Input: part model. Units: mm. Frame: model coordinates. Face numbers are marked on the shaded views. A direction names the side the tool comes from. Coordinates: 2 decimals unless noted, no trailing zeros. Order: outer loops, then holes, each group sorted by start corner. A loop starts at its lowest first (then second) coordinate and runs counter-clockwise, first axis right, second up. Notation, with made-up numbers: (4.25, -30.75) - (25.25, -30.75) arc R23 ccw to (25.25, 6.25) - close; hole circle Ø7 at (-2, -40). An arc over 180 degrees is marked (long way). Answer as CSV lines item,"result". Start each with the question number.
Item 1: Draft query along X for the marked faces 1, 2, 3 and 4. Return one class per face: +X half, -X half, draft (parallel to the pull), parting line (faces both ways), or undercut.
Item 2: Access query for the marked faces 5, 6 and 7. Directions: +Z, -Z, +X, -X, +Y, -Y. A direction counts if a zero-diameter tool reaches every point of the face in a straight line with its end or side. Return the directions, or none.
Item 3: Section B-B (x = -2). Output: boundary loops of the cut face in (y, z), and give its area (3 significant figures).
Item 4: Section A-A (z = -0.05). Output: boundary loops of the cut face in (x, y) (3 decimals), and give its area (3 significant figures).
Item 5: Material intervals for line 1 along X through (y, z) = (0, -0.5) (3 decimals); line 2 along X through (y, z) = (0, -0.05); line 3 along Y through (x, z) = (-0.7, 0.05) (3 decimals), sorted ascending.
Item 6: First-contact query: pin 1 (1 mm diameter, centred on x = 1.5, z = 1, fed in from -Y); pin 2 (2.5 mm diameter, centred on x = 0, y = 0, fed in from +Z) (3 decimals). Flat tips, straight axial feed; report the tip coordinate or a pass-through.
Item 7: Section C-C (z = 0.8). Output: boundary loops of the cut face in (x, y) (3 decimals).
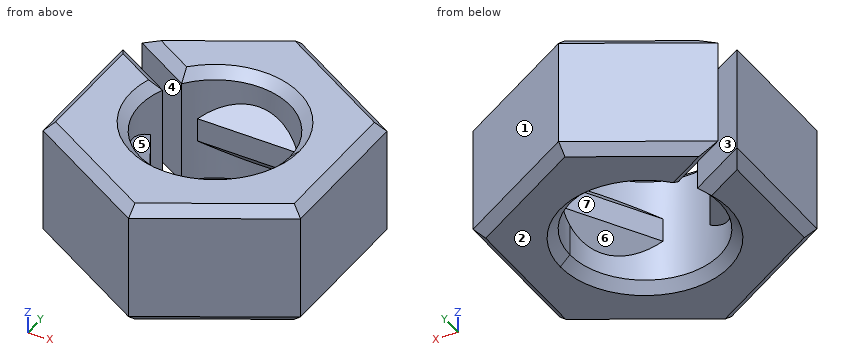
from build123d import *

# Parameters (mm, degrees)
SKETCH1_R                   = 1.575
BOSS_EXTRUDE1_DEPTH         = 1.3
CLIP_REACH                  = 6.324
CLIP_END_RADIUS             = 1.575
CLIP_DIRECTION_2_REACH      = 6.324
CLIP_DIRECTION_2_END_RADIUS = 1.575
CLIPS_X3_COUNT              = 3
SPLIT_2_DEPTH               = 5.324349662
SPLIT_2_DEPTH_BACK          = 5.324349662
DEBURS_SIZE                 = 0.2


with BuildPart() as part:
    # Sketch1 → Boss-Extrude1 (new, symmetric)
    with BuildSketch(Plane.XY):
        Polygon((2.7, -1.558845727), (2.7, 1.558845727), (0, 3.117691454), (-2.7, 1.558845727), (-2.7, -1.558845727), (0, -3.117691454), align=None)
        Circle(SKETCH1_R, mode=Mode.SUBTRACT)
    extrude(amount=BOSS_EXTRUDE1_DEPTH, both=True)

    # Clip: up to this cylinder (the profile starts inside it)
    clip_end = Plane(origin=(0, 0, 0), z_dir=(0, 0, -1)) * Cylinder(CLIP_END_RADIUS, 16.798, mode=Mode.PRIVATE)
    # Sketch3 → Clip (add, up to the surface)
    with BuildSketch(Plane(origin=(0, 0, 0), x_dir=(0, 0, -1), z_dir=(1, 0, 0)), mode=Mode.PRIVATE) as clip_sk1:
        Polygon((-0.65, 1.575), (0.65, 1.575), (0.25, 1.175), (-0.25, 1.175), align=None)
    clip_tool1 = extrude(clip_sk1.sketch, amount=CLIP_REACH, mode=Mode.PRIVATE) & clip_end
    clip = clip_tool1.solids().sort_by_distance((0, 1.40463, 0))[0]
    add(clip)

    # Clip direction 2: up to this cylinder (the profile starts inside it)
    clip_direction_2_end = Plane(origin=(0, 0, 0), z_dir=(0, 0, -1)) * Cylinder(CLIP_DIRECTION_2_END_RADIUS, 16.798, mode=Mode.PRIVATE)
    # Sketch3 → Clip direction 2 (add, up to the surface)
    with BuildSketch(Plane(origin=(0, 0, 0), x_dir=(0, 0, -1), z_dir=(1, 0, 0)), mode=Mode.PRIVATE) as clip_direction_2_sk1:
        Polygon((-0.65, 1.575), (0.65, 1.575), (0.25, 1.175), (-0.25, 1.175), align=None)
    clip_direction_2_tool1 = extrude(clip_direction_2_sk1.sketch, amount=-CLIP_DIRECTION_2_REACH, mode=Mode.PRIVATE) & clip_direction_2_end
    clip_direction_2 = clip_direction_2_tool1.solids().sort_by_distance((0, 1.40463, 0))[0]
    add(clip_direction_2)
    clip = clip + clip_direction_2  # both directions under the feature's name, for the pattern or mirror that repeats it

    # Clips x3: Clip ×3 about axis
    clips_x3_axis = Axis((0, 0, 0), (0, 0, 1))
    for i in range(1, CLIPS_X3_COUNT):
        add(clip.rotate(clips_x3_axis, i * 360 / CLIPS_X3_COUNT))

    # Sketch4 → Split 2 (cut, two sides: drawn at the far end of the back side and taken through both)
    with BuildSketch(Plane.XY.offset(-SPLIT_2_DEPTH_BACK)):
        Polygon((-2.8, 1.385640646), (-0.1, -0.173205081), (0.1, 0.173205081), (-2.6, 1.732050808), align=None)
    extrude(amount=SPLIT_2_DEPTH + SPLIT_2_DEPTH_BACK, mode=Mode.SUBTRACT)

    # Deburs
    deburs_edges = [part.edges().sort_by_distance(p)[0] for p in [
        (1.35, 2.33826859, 1.3),
        (-1.25, 2.396003617, 1.3),
        (-1.35, -2.33826859, 1.3),
        (-0.310025509, -1.544185605, 1.3),
        (1.35, -2.33826859, 1.3),
        (-0.310025509, -1.544185605, -1.3),
        (-2.7, -0.115470054, -1.3),
        (-2.7, -0.115470054, 1.3),
        (-2.076474085, 0.967912764, -1.3),
        (-1.876474085, 1.314322926, 1.3),
        (-1.876474085, 1.314322926, -1.3),
        (-2.076474085, 0.967912764, 1.3),
        (-1.35, -2.33826859, -1.3),
        (-1.25, 2.396003617, -1.3),
        (1.35, 2.33826859, -1.3),
        (2.7, 0, -1.3),
        (1.35, -2.33826859, -1.3),
        (2.7, 0, 1.3),
    ]]
    chamfer(deburs_edges, length=DEBURS_SIZE)


solid = part.part
Determined:
1,face 1,"+X half"
1,face 2,"draft"
1,face 3,"undercut"
1,face 4,"undercut"
2,face 5,"+Z"
2,face 6,"-Z"
2,face 7,"+Z, -Z"
3,outline,"(-1.96, -1.1) - (-1.73, -1.3) - (0.69, -1.3) - (0.92, -1.1) - (0.92, 1.1) - (0.69, 1.3) - (-1.73, 1.3) - (-1.96, 1.1) - close; (1.39, -1.1) - (1.62, -1.3) - (1.73, -1.3) - (1.96, -1.1) - (1.96, 1.1) - (1.73, 1.3) - (1.62, 1.3) - (1.39, 1.1) - close"
3,area,"8.82 mm^2"
4,outline,"(-2.7, -1.559) - (0, -3.118) - (2.7, -1.559) - (2.7, 1.559) - (0, 3.118) - (-2.5, 1.674) - (-1.253, 0.954) arc R1.575 cw to (-1.049, 1.175) - (1.049, 1.175) arc R1.575 cw to (1.542, 0.321) - (0.493, -1.496) arc R1.575 cw to (-0.493, -1.496) - (-1.542, 0.321) arc R1.575 cw to (-1.453, 0.608) - (-2.7, 1.328) - close"
4,area,"18.6 mm^2"
5,line 1,"x = -2.7 to -1.575, 1.575 to 2.7"
5,line 2,"x = -2.7 to -1.36, 1.36 to 2.7"
5,line 3,"y = -2.714 to -1.138, 1.175 to 2.714"
6,pin 1,"stops at y = -2.54"
6,pin 2,"stops at z = 0.325"
7,outline,"(-2.7, -1.559) - (0, -3.118) - (2.7, -1.559) - (2.7, 1.559) - (0, 3.118) - (-2.5, 1.674) - (-1.253, 0.954) arc R1.575 cw (long way) to (-1.453, 0.608) - (-2.7, 1.328) - close"
